Geometry: final body of the model. Coordinates: model frame, mm. A direction names the side the tool comes from. Round coordinates to 2 decimals unless told otherwise and drop trailing zeros. Write item = value, one per line. Start each with the question number.
Item 1: Draft query along X for faces 4 (the flat face through (-35, 15, 4)), 5 (the flat face through (26, 33, 1.5)), 6 (the flat face through (37, 30, 7.2)), 7 (the flat face through (18.35, 34, 6)). Return one class per face: pulls with the +X half, pulls with the -X half, needs draft (parallel to the pull), parting line crosses it, or undercut.
Item 2: First-contact query: pin 1 (5 mm diameter, centred on x = 1.5, y = 24.5, fed in from +Z); pin 2 (1.3 mm diameter, centred on y = 35, z = 3.5, fed in from -X); pin 3 (1.2 mm diameter, centred on x = 23.5, z = 2.5, fed in from +Y); pin 4 (6 mm diameter, centred on x = -18, y = 31, fed in from -Z). Flat tips, straight axial feed; report the tip coordinate or a pass-through.
Item 3: Line query: line 1 (Z direction, x = -22.5, y = 30.5); line 2 (X direction, y = 28.5, z = 3.25); line 3 (Y direction, x = -11.5, z = 4). Output: solid intervals per line, ascending. Write a range as from..to.
Item 4: Access query for faces 1 (the flat face through (-32.814, 1.149, 3.944)), 2 (the flat face through (0, 20.8, 5)), 3 (the flat face through (19.75, 35, 4)). Directions: +Z, -Z, +X, -X, +Y, -Y. A direction counts if a zero-diameter tool reaches every point of the face in a straight line with its end or side. Return the directions, or none.
from build123d import *

# Parameters (mm, degrees)
EXTRUDE1_DEPTH       = 8
SKETCH2_W            = 8.4
SKETCH2_H            = 4.7
EXTRUDE2_DEPTH       = 1.4
EXTRUDE3_DEPTH       = 4.2
EXTRUDE3_DEPTH_BACK  = 4.2
EXTRUDE4_DEPTH       = 4.2
EXTRUDE4_DEPTH_BACK  = 4.2
EXTRUDE5_DEPTH       = 1.7
EXTRUDE5_DEPTH_BACK  = 1.7
SKETCH5_W            = 2
SKETCH5_H            = 1
EXTRUDE6_DEPTH       = 8
EXTRUDE7_DEPTH       = 8
EXTRUDE8_DEPTH       = 5.8
EXTRUDE9_DEPTH       = 5.8
EXTRUDE10_DEPTH      = 2.5
EXTRUDE10_DEPTH_BACK = 2.5
EXTRUDE11_DEPTH      = 5
EXTRUDE11_DEPTH_BACK = 5
EXTRUDE12_DEPTH      = 1.5
EXTRUDE12_DEPTH_BACK = 1.5


with BuildPart() as part:
    # Sketch1 → Extrude1 (new body)
    with BuildSketch(Plane.XY):
        with BuildLine():
            Line((-34.824054735, -3.072067398), (-33.500260521, -6.190731128))
            ThreePointArc((-33.500260521, -6.190731128), (-33.131692653, -6.633885822), (-32.579755667, -6.8))
            Line((-32.579755667, -6.8), (-18.872283192, -6.8))
            ThreePointArc((-18.872283192, -6.8), (-17.083537757, -4.288835387), (-16.247280004, -1.321305957))
            Line((-16.247280004, -1.321305957), (-16.7, -1.2))
            Line((-16.7, -1.2), (-17.5, -1.2))
            Line((-17.5, -1.2), (-17.5, 0))
            Line((-17.5, 0), (-15.311743878, 0.191447604))
            ThreePointArc((-15.311743878, 0.191447604), (-14.485569293, 1.133519165), (-15.390706981, 2))
            Line((-15.390706981, 2), (-17.5, 2))
            Line((-17.5, 2), (-17.5, 5.3))
            ThreePointArc((-17.5, 5.3), (-16.882683432, 6.223879533), (-15.792893219, 6.007106781))
            Line((-15.792893219, 6.007106781), (-9.785786438, 0))
            Line((-9.785786438, 0), (17.5, 0))
            Line((17.5, 0), (17.5, -1.2))
            Line((17.5, -1.2), (16.741180955, -1.40332495))
            ThreePointArc((16.741180955, -1.40332495), (16.20664666, -1.760489348), (16, -2.369250777))
            Line((16, -2.369250777), (16, -3.5))
            ThreePointArc((16, -3.5), (16.292893219, -4.207106781), (17, -4.5))
            Line((17, -4.5), (19, -4.5))
            ThreePointArc((19, -4.5), (19.707106781, -4.207106781), (20, -3.5))
            Line((20, -3.5), (20, 6.1))
            ThreePointArc((20, 6.1), (20.058578644, 6.241421356), (20.2, 6.3))
            Line((20.2, 6.3), (48.5, 6.3))
            ThreePointArc((48.5, 6.3), (49.207106781, 6.592893219), (49.5, 7.3))
            Line((49.5, 7.3), (49.5, 23.635680518))
            ThreePointArc((49.5, 23.635680518), (49.366025404, 24.135680518), (49, 24.501705922))
            Line((49, 24.501705922), (35.551804172, 32.266025404))
            ThreePointArc((35.551804172, 32.266025404), (35.310623217, 32.365925826), (35.051804172, 32.4))
            Line((35.051804172, 32.4), (5.2, 32.4))
            ThreePointArc((5.2, 32.4), (4.990511031, 32.340755589), (4.843077314, 32.180571859))
            Line((4.843077314, 32.180571859), (4.2, 30.909449746))
            Line((4.2, 30.909449746), (4.2, 21.8))
            Line((4.2, 21.8), (-4.2, 21.8))
            Line((-4.2, 21.8), (-4.2, 30.909449746))
            Line((-4.2, 30.909449746), (-4.843077314, 32.180571859))
            ThreePointArc((-4.843077314, 32.180571859), (-4.990511031, 32.340755589), (-5.2, 32.4))
            Line((-5.2, 32.4), (-7.8, 32.4))
            ThreePointArc((-7.8, 32.4), (-8.157770876, 32.178885438), (-8.12, 31.76))
            Line((-8.12, 31.76), (-8, 31.6))
            ThreePointArc((-8, 31.6), (-7.996119463, 31.005244998), (-8.563727578, 30.827566639))
            Line((-8.563727578, 30.827566639), (-9.719017938, 31.227946689))
            ThreePointArc((-9.719017938, 31.227946689), (-10.189007481, 31.062306212), (-10.132842712, 30.567157288))
            Line((-10.132842712, 30.567157288), (-9.85, 30.284314575))
            Line((-9.85, 30.284314575), (-9.85, 29.4))
            Line((-9.85, 29.4), (-13, 29.4))
            Line((-13, 29.4), (-16.15, 29.4))
            Line((-16.15, 29.4), (-16.15, 30.284314575))
            Line((-16.15, 30.284314575), (-15.867157288, 30.567157288))
            ThreePointArc((-15.867157288, 30.567157288), (-15.810992519, 31.062306212), (-16.280982062, 31.227946689))
            Line((-16.280982062, 31.227946689), (-17.436272422, 30.827566639))
            ThreePointArc((-17.436272422, 30.827566639), (-18.003880537, 31.005244998), (-18, 31.6))
            Line((-18, 31.6), (-17.88, 31.76))
            ThreePointArc((-17.88, 31.76), (-17.842229124, 32.178885438), (-18.2, 32.4))
            Line((-18.2, 32.4), (-21.051804172, 32.4))
            ThreePointArc((-21.051804172, 32.4), (-21.310623217, 32.365925826), (-21.551804172, 32.266025404))
            Line((-21.551804172, 32.266025404), (-34.5, 24.790381057))
            ThreePointArc((-34.5, 24.790381057), (-34.866025404, 24.424355653), (-35, 23.924355653))
            Line((-35, 23.924355653), (-35, 6.3))
            Line((-35, 6.3), (-30.564941956, -4.148341984))
            ThreePointArc((-30.564941956, -4.148341984), (-31.474501075, -5.396338117), (-32.145272576, -4.005346482))
            ThreePointArc((-32.145272576, -4.005346482), (-32.121013363, -3.911579893), (-32.15911356, -3.822534638))
            Line((-32.15911356, -3.822534638), (-34.102040633, -1.664695515))
            ThreePointArc((-34.102040633, -1.664695515), (-35.366900567, -1.76337794), (-34.945835863, -2.960170899))
            ThreePointArc((-34.945835863, -2.960170899), (-34.872837521, -3.002941804), (-34.824054735, -3.072067398))
        make_face()
    extrude(amount=EXTRUDE1_DEPTH)

    # Sketch2 → Extrude2 (add)
    with BuildSketch(Plane.XY):
        with Locations((0, 24.15)):
            Rectangle(SKETCH2_W, SKETCH2_H)
    extrude(amount=EXTRUDE2_DEPTH)

    # Sketch3 → Extrude3 (cut, two sides: drawn at the far end of the back side and taken through both)
    with BuildSketch(Plane(origin=(0, 0, 0), x_dir=(0, 0, -1), z_dir=(1, 0, 0)).offset(-EXTRUDE3_DEPTH_BACK)):
        Polygon((-7.577350269, 21.8), (-7, 20.8), (-5.3, 20.8), (-4.722649731, 21.8), align=None)
    extrude(amount=EXTRUDE3_DEPTH + EXTRUDE3_DEPTH_BACK, mode=Mode.SUBTRACT)

    # Sketch4 → Extrude4 (cut, two sides: drawn at the far end of the back side and taken through both)
    with BuildSketch(Plane(origin=(0, 0, 0), x_dir=(0, 0, -1), z_dir=(1, 0, 0)).offset(-EXTRUDE4_DEPTH_BACK)):
        Polygon((-4.677350269, 21.8), (-4.1, 20.8), (-2.4, 20.8), (-1.822649731, 21.8), align=None)
    extrude(amount=EXTRUDE4_DEPTH + EXTRUDE4_DEPTH_BACK, mode=Mode.SUBTRACT)

    # Sketch5 → Extrude5 (cut, two sides: drawn at the far end of the back side and taken through both)
    with BuildSketch(Plane(origin=(0, 0, 0), x_dir=(0, 0, -1), z_dir=(1, 0, 0)).offset(-EXTRUDE5_DEPTH_BACK)):
        with Locations((-4.7, 21.3)):
            Rectangle(SKETCH5_W, SKETCH5_H)
    extrude(amount=EXTRUDE5_DEPTH + EXTRUDE5_DEPTH_BACK, mode=Mode.SUBTRACT)

    # Sketch6 → Extrude6 (add)
    with BuildSketch(Plane.XY):
        Polygon((3.25, 20.8), (4.2, 20.8), (4.2, 21.8), (3.827350269, 21.8), align=None)
    extrude(amount=EXTRUDE6_DEPTH)

    # Sketch7 → Extrude7 (add)
    with BuildSketch(Plane.XY):
        Polygon((-4.2, 21.8), (-4.2, 20.8), (-3.25, 20.8), (-3.827350269, 21.8), align=None)
    extrude(amount=EXTRUDE7_DEPTH)

    # Sketch8 → Cut-Revolve1 (revolve, cut)
    with BuildSketch(Plane.XY.offset(4), mode=Mode.PRIVATE) as cut_revolve1_sk:
        Polygon((42.127146997, 21.137401035), (39.269263165, 22.787401035), (42.184455543, 27.836662349), (42.184455543, 28.436662349), (45.302146997, 26.636662349), align=None)
    revolve(cut_revolve1_sk.sketch.rotate(Axis((45.302146997, 26.636662349, 4), (-0.4999999999999722, -0.8660254037844548, 0)), 180), axis=Axis((45.302146997, 26.636662349, 4), (-0.4999999999999722, -0.8660254037844548, 0)), mode=Mode.SUBTRACT)

    # Sketch9 → Cut-Revolve2 (revolve, cut)
    with BuildSketch(Plane.XY.offset(4), mode=Mode.PRIVATE) as cut_revolve2_sk:
        Polygon((-31.002146997, 26.80986743), (-27.884455543, 28.60986743), (-27.884455543, 28.00986743), (-24.969263165, 22.960606116), (-27.827146997, 21.310606116), align=None)
    revolve(cut_revolve2_sk.sketch.rotate(Axis((-27.827146997, 21.310606116, 4), (-0.49999999999997385, 0.8660254037844538, 0)), 180), axis=Axis((-27.827146997, 21.310606116, 4), (-0.49999999999997385, 0.8660254037844538, 0)), mode=Mode.SUBTRACT)

    # Sketch10 → Extrude8 (cut)
    with BuildSketch(Plane.XY.offset(1.4)):
        Polygon((34.212951043, 30.729611541), (38.646064357, 28.170152376), (39.889488223, 29.761662349), (34.953143422, 32.611662349), (34.80082943, 31.747846776), align=None)
    extrude(amount=EXTRUDE8_DEPTH, mode=Mode.SUBTRACT)

    # Sketch11 → Extrude9 (cut)
    with BuildSketch(Plane.XY.offset(1.4)):
        Polygon((-25.589488223, 29.93486743), (-24.346064357, 28.343357457), (-19.912951043, 30.902816622), (-20.50082943, 31.921051857), (-20.653143422, 32.78486743), align=None)
    extrude(amount=EXTRUDE9_DEPTH, mode=Mode.SUBTRACT)

    # Sketch12 → Extrude10 (add, two sides: drawn at the far end of the back side and taken through both)
    with BuildSketch(Plane.XY.offset(4).offset(-EXTRUDE10_DEPTH_BACK)):
        with BuildLine():
            Line((10.15, 31.65), (31.3, 31.65))
            Line((31.3, 31.65), (31.3, 32.9))
            Line((31.3, 32.9), (32, 33.087564435))
            Line((32, 33.087564435), (32, 35.9))
            Line((32, 35.9), (32.4, 35.9))
            Line((32.4, 35.9), (32.4, 36.4))
            ThreePointArc((32.4, 36.4), (32.253553391, 36.753553391), (31.9, 36.9))
            Line((31.9, 36.9), (27.270332061, 36.9))
            Line((27.270332061, 36.9), (26.05, 35.157185199))
            Line((26.05, 35.157185199), (26.05, 33.2))
            Line((26.05, 33.2), (18.35, 33.2))
            Line((18.35, 33.2), (18.35, 35.157185199))
            Line((18.35, 35.157185199), (17.129667939, 36.9))
            Line((17.129667939, 36.9), (16.3, 36.9))
            Line((16.3, 36.9), (16.3, 32.4))
            Line((16.3, 32.4), (12.949038106, 32.4))
            ThreePointArc((12.949038106, 32.4), (11.261771432, 33.098888739), (10.15, 31.65))
        make_face()
    extrude(amount=EXTRUDE10_DEPTH + EXTRUDE10_DEPTH_BACK)

    # Sketch13 → Extrude11 (add, two sides: drawn at the far end of the back side and taken through both)
    with BuildSketch(Plane(origin=(22.2, 0, 0), x_dir=(0, 0, -1), z_dir=(1, 0, 0)).offset(-EXTRUDE11_DEPTH_BACK)):
        with BuildLine():
            Line((-5.15, 34.026794919), (-5, 33.940192379))
            Line((-5, 33.940192379), (-5, 33.2))
            Line((-5, 33.2), (-3, 33.2))
            Line((-3, 33.2), (-3, 33.940192379))
            Line((-3, 33.940192379), (-2.85, 34.026794919))
            ThreePointArc((-2.85, 34.026794919), (-2.756642553, 34.14888349), (-2.777468634, 34.301157934))
            Line((-2.777468634, 34.301157934), (-3.482405902, 35.503473803))
            ThreePointArc((-3.482405902, 35.503473803), (-4, 35.8), (-4.517594098, 35.503473803))
            Line((-4.517594098, 35.503473803), (-5.222531366, 34.301157934))
            ThreePointArc((-5.222531366, 34.301157934), (-5.243357447, 34.14888349), (-5.15, 34.026794919))
        make_face()
    extrude(amount=EXTRUDE11_DEPTH + EXTRUDE11_DEPTH_BACK)

    # Sketch14 → Extrude12 (cut, two sides: drawn at the far end of the back side and taken through both)
    with BuildSketch(Plane.XY.offset(4).offset(-EXTRUDE12_DEPTH_BACK)):
        Polygon((17.129667939, 36.9), (18.25, 35.3), (19.32225346, 35.8), (19.75, 35.8), (19.75, 34.2), (21.15, 34.2), (21.15, 35.8), (23.25, 35.8), (23.25, 34.2), (24.65, 34.2), (24.65, 35.8), (25.07774654, 35.8), (26.15, 35.3), (27.270332061, 36.9), (22.2, 36.9), align=None)
    extrude(amount=EXTRUDE12_DEPTH + EXTRUDE12_DEPTH_BACK, mode=Mode.SUBTRACT)


solid = part.part
Taken from the geometry:
q1.face_4 = pulls with the -X half
q1.face_5 = needs draft
q1.face_6 = undercut
q1.face_7 = undercut
q2.pin_1 = 1.4
q2.pin_2 = 16.3
q2.pin_3 = 34.76
q2.pin_4 = 0
q3.line_1 = 0..1.4, 7.2..8
q3.line_2 = -27.95..-24.47, -24.07..-4.2, 4.2..38.07, 38.9..42.07
q3.line_3 = 1.71..29.4
q4.face_1 = +Z, -Z
q4.face_2 = +Y
q4.face_3 = +Z, -Z, +Y
